Here's the drawing with two shaded views (mm, measured from the low corner). I have some questions. Coordinates: 2 decimals unless noted, no trailing zeros. Write each loop counter-clockwise with the first axis right and the second up, starting at its lowest first coordinate (ties: lowest second). Pieces come first, ordered by that corner, then holes.
Item 1: If we section it at A-A (x = 99): Please give me the cut outline in (y, z), then the cut area to 3 significant figures.
Item 2: If I drill on line 1 (Z direction, x = 37.5, y = 82); line 2 (Y direction, x = 60.5, z = 15); line 3 (Y direction, x = 117.5, z = 2) (1 decimal), over which ranges is the centre line in solid material (lowest first)?
Item 3: If we section it at B-B (y = 83): Please give me the cut outline in (x, z).
Item 4: I'm going to push flat-ended pins straight in: pin 1 Ø12 at (y, z) = (61.5, 12) entering from +X; pin 2 Ø0.8 at (x, z) = (97, 40.5) entering from +Y; pin 3 Ø6 at (y, z) = (44.5, 25.5) entering from -X (1 decimal); pin 4 Ø10 at (x, y) = (52.5, 21) entering from -Z. Where does each tip first touch, or does it pass through?
Item 5: If we section it at C-C (z = 23.5): Please give me the cut outline in (x, y), then the cut area to 3 significant figures.
Item 6: If we section it at D-D (y = 30.5): Please give me the cut outline in (x, z) (1 decimal).
Item 7: We'd pull the mould along Z, two halves only. Please class the marked faces 1, 2, 3 and 4: +Z half, -Z half, draft (parallel to the pull), parting line (faces both ways), or undercut.
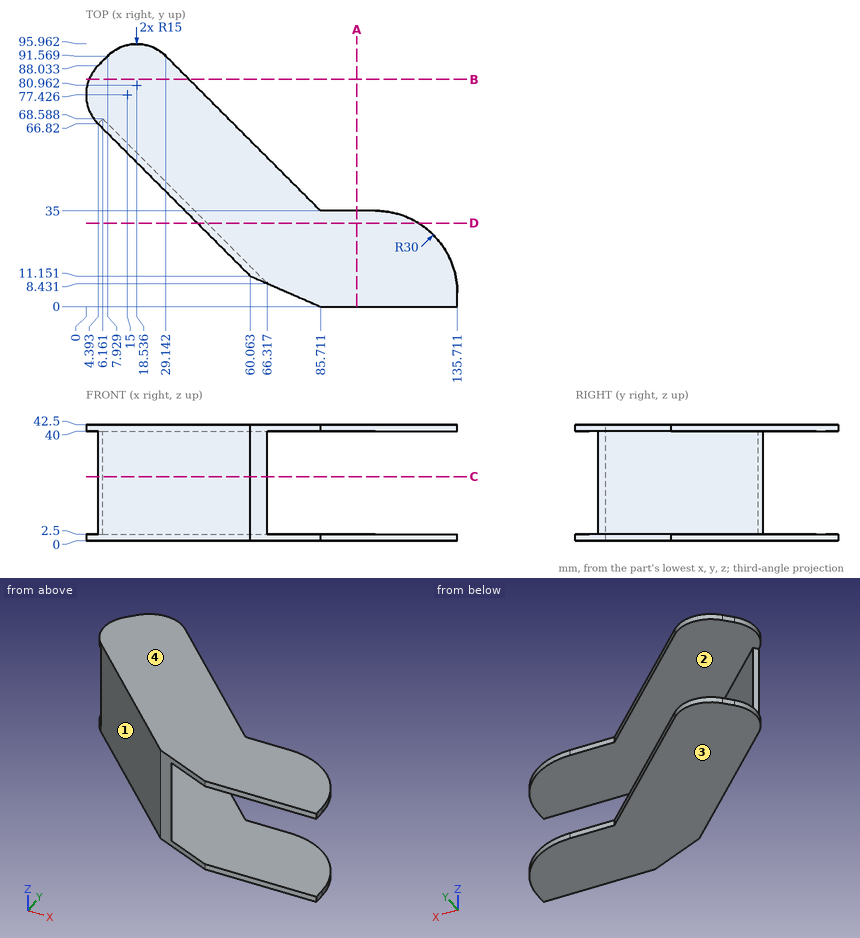
Answer list:
1. outline: (0, 0) - (35, 0) - (35, 2.5) - (0, 2.5) - close; (0, 40) - (35, 40) - (35, 42.5) - (0, 42.5) - close
1. area: 175 mm2
2. line 1: z = 0 to 2.5, 40 to 42.5
2. line 2: y = 10.96 to 14.25
2. line 3: y = 0 to 32.6
3. outline: (1.07, 0) - (37.71, 0) - (37.71, 2.5) - (1.07, 2.5) - close; (1.07, 40) - (37.71, 40) - (37.71, 42.5) - (1.07, 42.5) - close
4. pin 1: stops at x = 19.25
4. pin 2: stops at y = 35
4. pin 3: stops at x = 23.7
4. pin 4: stops at z = 0
5. outline: (4.39, 66.82) - (60.06, 11.15) - (66.32, 8.43) - (6.16, 68.59) - close
5. area: 205 mm2
6. outline: (40.7, 0) - (121.5, 0) - (121.5, 2.5) - (44.2, 2.5) - (44.2, 40) - (121.5, 40) - (121.5, 42.5) - (40.7, 42.5) - close
7. face 1: draft
7. face 2: undercut
7. face 3: -Z half
7. face 4: +Z half
